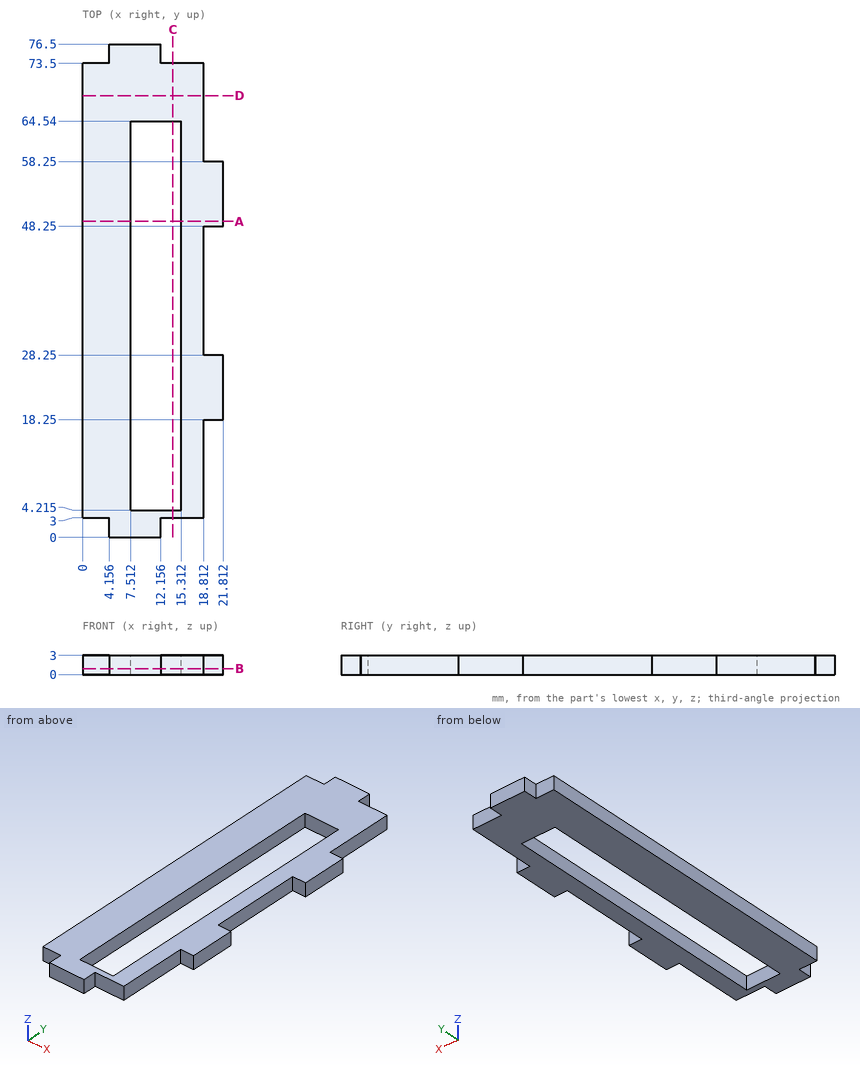
Print and shaded views of the part. All mm, measured from the part's lowest x, y and z. Coordinates: 2 decimals unless noted, no trailing zeros. Order: outer loops, then holes, each group sorted by start corner. A loop starts at its lowest first (then second) coordinate and runs counter-clockwise, first axis right, second up.
(1) Slice it at D-D, the plane y = 68.5. Write the cut outline in (x, z).
Check sheet entries:
outline: (0, 0) - (18.81, 0) - (18.81, 3) - (0, 3) - close
(2) Slice it at B-B, the plane z = 0.95. Write the cut outline in (x, y) (3 decimals), and give its area (3 significant figures).
Check sheet entries:
outline: (0, 3) - (4.156, 3) - (4.156, 0) - (12.156, 0) - (12.156, 3) - (18.812, 3) - (18.812, 18.25) - (21.812, 18.25) - (21.812, 28.25) - (18.812, 28.25) - (18.812, 48.25) - (21.812, 48.25) - (21.812, 58.25) - (18.812, 58.25) - (18.812, 73.5) - (12.156, 73.5) - (12.156, 76.5) - (4.156, 76.5) - (4.156, 73.5) - (0, 73.5) - close; hole (7.512, 4.215) - (15.312, 4.215) - (15.312, 64.54) - (7.512, 64.54) - close
area: 964 mm2
(3) Probe L1, parallel to X at y = 60, z = 0.5; L2, parallel to Y at x = 8, z = 1.5 (3 decimals); L3, parallel to Y at x = 20, z = 2.65. List the from-to ranges inside material, lowest first.
Check sheet entries:
L1: x = 0 to 7.51, 15.31 to 18.81
L2: y = 0 to 4.215, 64.54 to 76.5
L3: y = 18.25 to 28.25, 48.25 to 58.25
(4) Pin check, flat tips, straight feed: pin 1 Ø1.5 at (x, z) = (13, 2) entering from -Y; pin 2 Ø1 at (y, z) = (39.5, 0.5) entering from +X; pin 3 Ø1.5 at (y, z) = (2, 1.5) entering from +X. Stop position of each tip, or through.
Check sheet entries:
pin 1: stops at y = 3
pin 2: stops at x = 18.81
pin 3: stops at x = 12.16
(5) Slice it at A-A, the plane y = 49. Write the cut outline in (x, z), and give its area (3 significant figures).
Check sheet entries:
outline: (0, 0) - (7.51, 0) - (7.51, 3) - (0, 3) - close; (15.31, 0) - (21.81, 0) - (21.81, 3) - (15.31, 3) - close
area: 42.0 mm2
(6) Slice it at C-C, the plane x = 14. Write the cut outline in (y, z) (3 decimals), and give its area (3 significant figures).
Check sheet entries:
outline: (3, 0) - (4.215, 0) - (4.215, 3) - (3, 3) - close; (64.54, 0) - (73.5, 0) - (73.5, 3) - (64.54, 3) - close
area: 30.5 mm2
